Read the model definition and answer for the solid it produces. Units are mm, in the model's axes. Coordinates: 2 decimals unless noted, no trailing zeros. Write each loop counter-clockwise with the first axis right and the second up, starting at its lowest first coordinate (ties: lowest second). Pieces come first, ordered by that corner, then holes. Notation, with made-up numbers: (68.25, -4.5) - (121.25, -4.5) arc R16 ccw to (121.25, 22.5) - close; hole circle Ø8 at (64.25, 22.25). An arc over 180 degrees is marked (long way). Use a Markdown table: item, result.
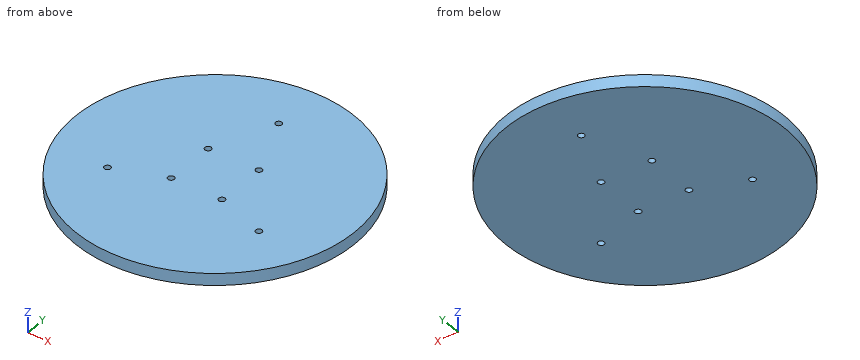
Autodesk Inventor part; units mm, degrees
ref_plane "YZ Plane" through (0, 0, 0) normal (1, 0, 0) x (0, 1, 0)
ref_plane "XZ Plane" through (0, 0, 0) normal (0, 1, 0) x (-1, 0, 0)
ref_plane "XY Plane" through (0, 0, 0) normal (0, 0, 1) x (1, 0, 0)
sketch "Skizze1" plane through (0, 0, 0) normal (0, 0, 1) x (1, 0, 0)
  circle A0 centre (0, 0) radius 175
  dimension "d0" = 350
extrude "Extrusion1" add sketch "Skizze1" against normal blind 15
sketch "Skizze2" plane through (0, 0, 0) normal (0, 0, 1) x (1, 0, 0)
  line L0 (-32, 32) -> (32, 32)
  line L1 (32, 32) -> (32, -32)
  line L2 (32, -32) -> (-32, -32)
  line L3 (-32, -32) -> (-32, 32)
  line L4 (-32, 32) -> (32, -32) construction
  line L5 (32, 32) -> (-32, -32) construction
  circle A0 centre (0, 0) radius 110
  line L6 (0, -245) -> (0, 245)
  point P0 (0, 110)
  point P1 (-95.2628, -55)
  point P2 (95.2628, -55)
  dimension "d3" = 64
  dimension "d4" = 64
  dimension "d5" = 220
hole "Bohrung1" at (32, 32, 0) at (-32, 32, 0) at (-32, -32, 0) at (32, -32, 0) at (0, 110, 0) at (-95.2628, -55, 0) at (95.2628, -55, 0) direction (0, 0, -1) diameter 8 end through all
properties part number "Verbindungsplatte_Staender"
(1) A cutting plane is placed at D-D, the plane z = -8.25. Write down the section's boundary in (x, y).
Report:
| item | result |
|---|---|
| outline | circle Ø350 at (0, 0); hole circle Ø8 at (-95.26, -55); hole circle Ø8 at (-32, -32); hole circle Ø8 at (-32, 32); hole circle Ø8 at (0, 110); hole circle Ø8 at (32, -32); hole circle Ø8 at (32, 32); hole circle Ø8 at (95.26, -55) |
(2) Straight lines are drawn through the part: L1, parallel to Y at x = 0, z = -8.5; L2, parallel to Y at x = -32, z = -10.5; L3, parallel to X at y = -55, z = -4.5. For each, find the intervals that lie inside material, in ascending order.
Report:
| item | result |
|---|---|
| L1 | y = -175 to 106, 114 to 175 |
| L2 | y = -172.05 to -36, -28 to 28, 36 to 172.05 |
| L3 | x = -166.13 to -99.26, -91.26 to 91.26, 99.26 to 166.13 |
(3) A cutting plane is placed at A-A, the plane y = 110. Write down the section's boundary in (x, z), and give its area (3 significant figures).
Report:
| item | result |
|---|---|
| outline | (-136.11, -15) - (-4, -15) - (-4, 0) - (-136.11, 0) - close; (4, -15) - (136.11, -15) - (136.11, 0) - (4, 0) - close |
| area | 3,960 mm² |
(4) Each of these flat-tipped pins is pushed along its axis until it touches: P1, Ø3, axis at y = 77, z = -5.5, coming from the -X side; P2, Ø4, axis at y = 71.5, z = -10, coming from the +X side; P3, Ø7, axis at x = 0, y = 110, coming from the -Z side; P4, Ø4, axis at x = 133, z = -12, coming from the +Y side. Where does it stop, or does it pass through?
Report:
| item | result |
|---|---|
| P1 | stops at x = -157.88 |
| P2 | stops at x = 160.61 |
| P3 | passes through |
| P4 | stops at y = 116.03 |
(5) A cutting plane is placed at B-B, the plane x = 32. Write down the section's boundary in (y, z).
Report:
| item | result |
|---|---|
| outline | (-172.05, -15) - (-36, -15) - (-36, 0) - (-172.05, 0) - close; (-28, -15) - (28, -15) - (28, 0) - (-28, 0) - close; (36, -15) - (172.05, -15) - (172.05, 0) - (36, 0) - close |
